Can you work these out from the model? Positions are in its coordinate system, mm. A direction names the side the tool comes from. Coordinates: 2 decimals unless noted, no trailing zeros. Loops run counter-clockwise (first coordinate to the right, second up) from the corner with the lowest first, then second, coordinate; pieces in that order, holes last. Notation, with made-up numbers: (9, -11) -> (24, -11) arc R26 ccw to (24, 15) -> close; hole circle Ø3 at (-24, 42.25). An arc over 180 degrees is marked (long way). Put each result on its own line as item: value. Start each with the question number.
Item 1: Please list where these lines run through material, in increasing order: L1, parallel to X at y = 6, z = -54; L2, parallel to X at y = 6.75, z = -8; L3, parallel to Y at x = -2.5, z = -28. Write a range as from..to.
Item 2: We'd pull the mould along X, two halves only. Please class faces 1 (the flat face through (-29.324, 8, -29)), 2 (the flat face through (3, 11.02, -52)), 3 (the flat face through (-9, 3, -59.3)), 4 (the cylindrical face through (10.134, -0.429, -29.235)): pulls with the +X half, pulls with the -X half, needs draft (parallel to the pull), parting line crosses it, or undercut.
Item 3: Will these pins go through, and if not, where does the flat tip stop? P1, Ø3.5, axis at x = -12.62, z = -51.5, coming from the +Y side; P2, Ø1.1, axis at x = -0.5, z = -54.5, coming from the +Y side; P3, Ø1, axis at x = 6, z = -15.5, coming from the +Y side.
Item 4: If we section it at B-B on y = 4.25: Please give me the cut outline in (x, z).
Item 5: For faces 5 (the flat face through (-24, 1, -29)), 6 (the flat face through (-20.624, 8, -51)), 7 (the flat face through (-5, 6, -46.3)), 8 (the flat face through (-5, 7, -55.3)), 9 (the cylindrical face through (-8.75, 11.53, -52.97)), which set-ups out of +Z, -Z, +X, -X, +Y, -Y let a thin tool reach every point of the face, with its end or its side?
Item 6: If we section it at D-D on x = 12: Please give me the cut outline in (y, z), plus the area to 3 significant figures.
Item 7: If we section it at A-A on y = 13.25: Please give me the cut outline in (x, z), plus the area to 3 significant figures.
Item 8: If we section it at C-C on z = -11.5: Please give me the cut outline in (x, y).
```python
from build123d import *

# Parameters (mm, degrees)
EXTRUDE_THIN1_DEPTH = 59.3
SKETCH2_W           = 44.2
SKETCH2_H           = 59.3
EXTRUDE1_DEPTH      = 1.6
EXTRUDE2_DEPTH      = 30.5
SKETCH4_R           = 1.85
EXTRUDE3_DEPTH      = 1.5
SKETCH6_R           = 1.85
EXTRUDE4_DEPTH      = 0.5
SKETCH8_W           = 0.615121557
SKETCH8_H           = 3.349209548
EXTRUDE5_DEPTH      = 0.4
LPATTERN1_COUNT     = 6
LPATTERN1_PITCH     = 5


with BuildPart() as part:
    # Sketch1 → Extrude-Thin1 (new body)
    with BuildSketch(Plane.XY):
        with BuildLine():
            Line((-28.323886885, 14), (-28.323886885, 2.9))
            ThreePointArc((-28.323886885, 2.9), (-28.060282988, 2.263603897), (-27.423886885, 2))
            Line((-27.423886885, 2), (-21.223886885, 2))
            ThreePointArc((-21.223886885, 2), (-20.587490782, 1.736396103), (-20.323886885, 1.1))
            Line((-20.323886885, 1.1), (-20.323886885, 0.9))
            ThreePointArc((-20.323886885, 0.9), (-20.060282988, 0.263603897), (-19.423886885, 0))
            Line((-19.423886885, 0), (8.776113115, 0))
            ThreePointArc((8.776113115, 0), (9.412509218, 0.263603897), (9.676113115, 0.9))
            Line((9.676113115, 0.9), (9.676113115, 1.1))
            ThreePointArc((9.676113115, 1.1), (9.939717012, 1.736396103), (10.576113115, 2))
            Line((10.576113115, 2), (16.776113115, 2))
            ThreePointArc((16.776113115, 2), (17.412509218, 2.263603897), (17.676113115, 2.9))
            Line((17.676113115, 2.9), (17.676113115, 14))
            Line((17.676113115, 14), (18.676113115, 14))
            Line((18.676113115, 14), (18.676113115, 2.9))
            ThreePointArc((18.676113115, 2.9), (18.119615999, 1.556497116), (16.776113115, 1))
            Line((16.776113115, 1), (10.676113115, 1))
            Line((10.676113115, 1), (10.676113115, 0.9))
            ThreePointArc((10.676113115, 0.9), (10.119615999, -0.443502884), (8.776113115, -1))
            Line((8.776113115, -1), (-19.423886885, -1))
            ThreePointArc((-19.423886885, -1), (-20.767389769, -0.443502884), (-21.323886885, 0.9))
            Line((-21.323886885, 0.9), (-21.323886885, 1))
            Line((-21.323886885, 1), (-27.423886885, 1))
            ThreePointArc((-27.423886885, 1), (-28.767389769, 1.556497116), (-29.323886885, 2.9))
            Line((-29.323886885, 2.9), (-29.323886885, 14))
            Line((-29.323886885, 14), (-28.323886885, 14))
        make_face()
    extrude(amount=-EXTRUDE_THIN1_DEPTH)



with BuildPart() as body_2:
    # Sketch2 → Extrude1 (new body)
    with BuildSketch(Plane(origin=(0, 2, 0), x_dir=(1, 0, 0), z_dir=(0, 1, 0))):
        with Locations((-5.323886885, 29.65)):
            Rectangle(SKETCH2_W, SKETCH2_H)
    extrude(amount=EXTRUDE1_DEPTH)


with BuildPart() as part_1:
    add(part.part)

    add(body_2.part)  # Extrude2 merges body 2
    # Sketch3 → Extrude2 (add)
    with BuildSketch(Plane.ZY.offset(-9.876113115)):
        Polygon((-55.3, 3.6), (-46.3, 3.6), (-46.3, 7.6), (-49.003148697, 12.020138766), (-54.003148697, 12.020138766), (-54.3, 9.6), (-55.3, 9.6), align=None)
    extrude(amount=EXTRUDE2_DEPTH)

    # Sketch4 → Extrude3 (cut)
    with BuildSketch(Plane(origin=(0, 12.020138766, 0), x_dir=(1, 0, 0), z_dir=(0, 1, 0))):
        with Locations(Location((-17.623886885, 51.503148697, 0), (0, 0, 270))):
            Circle(SKETCH4_R)
    extrude3 = extrude(amount=-EXTRUDE3_DEPTH, mode=Mode.SUBTRACT)

    # Sketch6 → Extrude4 (add)
    with BuildSketch(Plane(origin=(0, 10.520138766, 0), x_dir=(1, 0, 0), z_dir=(0, 1, 0))):
        with Locations(Location((-17.623886885, 51.503148697, 0), (0, 0, 270))):
            Circle(SKETCH6_R)
    extrude4 = extrude(amount=EXTRUDE4_DEPTH)

    # Sketch8 → Extrude5 (cut)
    with BuildSketch(Plane(origin=(0, 11.020138766, 0), x_dir=(1, 0, 0), z_dir=(0, 1, 0))):
        with Locations((-17.623886885, 51.503148697)):
            Rectangle(SKETCH8_W, SKETCH8_H)
    extrude5 = extrude(amount=-EXTRUDE5_DEPTH, mode=Mode.SUBTRACT)

    # LPattern1: Extrude3, Extrude4, Extrude5 ×6
    with Locations(*[(i * LPATTERN1_PITCH, 0, 0) for i in range(1, LPATTERN1_COUNT)]):
        add(extrude3, mode=Mode.SUBTRACT)
        add(extrude4)
        add(extrude5, mode=Mode.SUBTRACT)


solid = part_1.part
```
Solutions:
1. L1: -29.32..-28.32, -20.62..9.88, 17.68..18.68
1. L2: -29.32..-28.32, 17.68..18.68
1. L3: -1..0, 2..3.6
2. face 1: pulls with the -X half
2. face 2: undercut
2. face 3: needs draft
2. face 4: pulls with the +X half
3. P1: y = 11.02
3. P2: y = 12.02
3. P3: y = 3.6
4. outline: (-29.32, -59.3) -> (-28.32, -59.3) -> (-28.32, 0) -> (-29.32, 0) -> close; (-20.62, -55.3) -> (9.88, -55.3) -> (9.88, -46.3) -> (-20.62, -46.3) -> close; (17.68, -59.3) -> (18.68, -59.3) -> (18.68, 0) -> (17.68, 0) -> close
5. face 5: +Z, -Z, -X, -Y
5. face 6: +Z, -Z, +Y
5. face 7: +Z, +Y
5. face 8: -Z, +Y
5. face 9: +Y
6. outline: (1, -59.3) -> (3.6, -59.3) -> (3.6, 0) -> (1, 0) -> close
6. area: 154 mm^2
7. outline: (-29.32, -59.3) -> (-28.32, -59.3) -> (-28.32, 0) -> (-29.32, 0) -> close; (17.68, -59.3) -> (18.68, -59.3) -> (18.68, 0) -> (17.68, 0) -> close
7. area: 119 mm^2
8. outline: (-29.32, 2.9) arc R1.9 ccw to (-27.42, 1) -> (-21.32, 1) -> (-21.32, 0.9) arc R1.9 ccw to (-19.42, -1) -> (8.78, -1) arc R1.9 ccw to (10.68, 0.9) -> (10.68, 1) -> (16.78, 1) arc R1.9 ccw to (18.68, 2.9) -> (18.68, 14) -> (17.68, 14) -> (17.68, 2.9) arc R0.9 cw to (16.78, 2) -> (16.78, 3.6) -> (-27.42, 3.6) -> (-27.42, 2) arc R0.9 cw to (-28.32, 2.9) -> (-28.32, 14) -> (-29.32, 14) -> close; hole (-21.22, 2) arc R0.9 cw to (-20.32, 1.1) -> (-20.32, 0.9) arc R0.9 ccw to (-19.42, 0) -> (8.78, 0) arc R0.9 ccw to (9.68, 0.9) -> (9.68, 1.1) arc R0.9 cw to (10.58, 2) -> close
